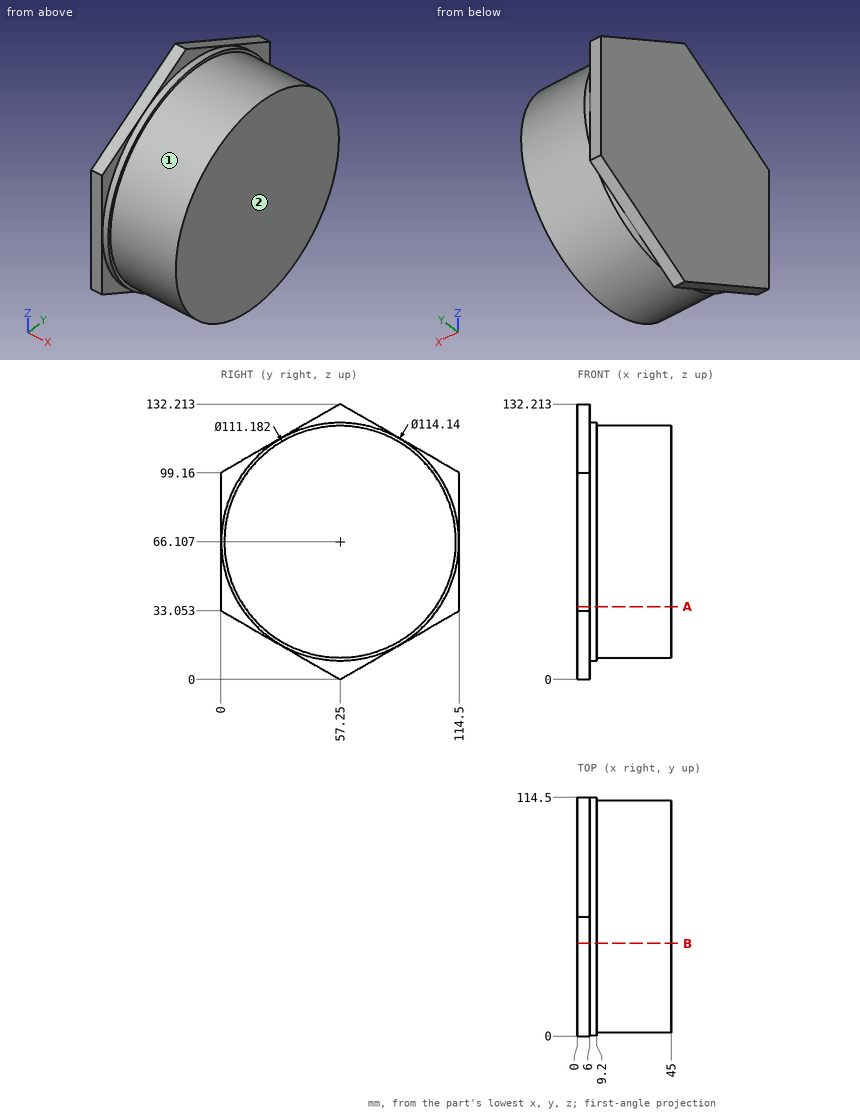
Design review of the part shown in the three views and the two pictorial views. Dimensions are in mm from the part's minimum x, y and z. A direction names the side the tool comes from. Round coordinates to 2 decimals unless told otherwise and drop trailing zeros. Write each loop counter-clockwise with the first axis right and the second up, starting at its lowest first coordinate (ties: lowest second). Pieces come first, ordered by that corner, then holes.
Item 1: Wall thickness on L1, parallel to X at y = 56, z = 9; L2, parallel to Y at x = 21, z = 96; L3, parallel to Z at x = 5, y = 59.5 (1 decimal): over which ranges is each line inside the solid? List them lowest first.
Item 2: For pin 1 Ø8 at (x, y) = (12, 93.5) entering from +Z; pin 2 Ø5 at (x, y) = (35, 51.5) entering from +Z; pin 3 Ø3 at (x, z) = (17.5, 31.5) entering from -Y, all flat-tipped, find the tip position at first contact; note any pin that passes through.
Item 3: Consider section B-B on y = 44.5. Give the boundary of the cut face in (x, z) (1 decimal).
Item 4: For the marked faces 1 and 2, list the 3-axis set-ups (+Z, -Z, +X, -X, +Y, -Y) from which the entire face can be reached by the end or side of a thin tool; tool diameter is ignored.
Item 5: Consider section A-A on z = 35. Give the boundary of the cut face in (x, y), and give its area (3 significant figures).
Check values:
1. L1: x = 0 to 6
1. L2: y = 10.38 to 104.12
1. L3: z = 1.3 to 130.9
2. pin 1: stops at z = 112.39
2. pin 2: stops at z = 121.6
2. pin 3: stops at y = 12.59
3. outline: (0, 7.4) - (6, 7.4) - (6, 10.5) - (9.2, 10.5) - (9.2, 12) - (45, 12) - (45, 120.2) - (9.2, 120.2) - (9.2, 121.7) - (6, 121.7) - (6, 124.9) - (0, 124.9) - close
4. face 1: +X
4. face 2: +Z, -Z, +X, +Y, -Y
5. outline: (0, 0) - (6, 0) - (6, 9.4) - (9.2, 9.4) - (9.2, 11.18) - (45, 11.18) - (45, 103.32) - (9.2, 103.32) - (9.2, 105.1) - (6, 105.1) - (6, 114.5) - (0, 114.5) - close
5. area: 4,290 mm2
